Autodesk Inventor part; units mm, degrees
ref_plane "YZ Plane" through (0, 0, 0) normal (1, 0, 0) x (0, 1, 0)
ref_plane "XZ Plane" through (0, 0, 0) normal (0, 1, 0) x (-1, 0, 0)
ref_plane "XY Plane" through (0, 0, 0) normal (0, 0, 1) x (1, 0, 0)
sketch "Sketch1" plane through (0, 0, 0) normal (0, 0, 1) x (1, 0, 0)
  line L0 (0, 0) -> (37.6224, 0)
  line L1 (0, 35) -> (0, 48)
  line L2 (0, 48) -> (12.1, 50)
  line L3 (12.1, 50) -> (13.1, 50)
  line L4 (0, 35) -> (11, 34.0376)
  line L5 (11, 34.0376) -> (11, 8)
  line L6 (11, 8) -> (-1, 8)
  line L7 (-1, 8) -> (-1, 0)
  line L8 (13.1, 50) -> (13.1, 0)
  line L9 (-1, 0) -> (13.1, 0)
  line L10 (26.2, 35) -> (26.2, 48)
  line L11 (26.2, 48) -> (14.1, 50)
  line L12 (14.1, 50) -> (13.1, 50)
  line L13 (26.2, 35) -> (15.2, 34.0376)
  line L14 (15.2, 34.0376) -> (15.2, 8)
  line L15 (15.2, 8) -> (27.2, 8)
  line L16 (27.2, 8) -> (27.2, 0)
  line L17 (27.2, 0) -> (13.1, 0)
  point P0 (26.2, 0)
  dimension "d0" = 100
  dimension "d2" = 1
  dimension "d3" = 13
  dimension "d4" = 13.1
  dimension "d5" = 11
  dimension "d6" = 95
  dimension "d7" = 16
  dimension "d8" = 12
  dimension "d9" = 48
revolve "Revolution1" add sketch "Sketch1" angle 360 about axis through (0, 0, 0) along (1, 0, 0)
hole "Hole1" at (27.2, 0, 0) direction (-1, 0, 0) diameter 8 end through all
fillet "Fillet1" radius 4 2 edges at (15.2, -8, 0) (11, -8, 0)
fillet "Fillet2" radius 2 2 edges at (15.2, -34.0376, 0) (11, -34.0376, 0)
properties part number "Hjul"
Build history of the part. All positions in model axes, mm. A direction names the side the tool comes from. Give positions to 0.01 mm unless a question says otherwise; leave off trailing zeros. Loops run counter-clockwise (first coordinate to the right, second up) from the corner with the lowest first, then second, coordinate; pieces in that order, holes last.
1) Band-saw the part on A-A on x = 24.5. List the corners of the cut face in (y, z), then the cut area to 3 significant figures.
Values follow:
outline: circle Ø96.56 at (0, 0); circle Ø16 at (0, 0); hole circle Ø69.7 at (0, 0); hole circle Ø8 at (0, 0)
area: 3,660 mm2
2) Two-plate mould, pull along Y, no slides. Class faces 4 (the face through (15.2, 14, 0)), 5 (the face through (0, 3.3, -35.3)), 6 (the face through (13.11, 47.69, 15.02)): released by +Y, released by -Y, zero draft, split by the parting line, or undercut.
Values follow:
face 4: undercut
face 5: zero draft
face 6: split by the parting line
3) Band-saw the part on B-B on x = 2.75. List the corners of the cut face in (y, z).
Values follow:
outline: circle Ø96.91 at (0, 0); circle Ø16 at (0, 0); hole circle Ø69.52 at (0, 0); hole circle Ø8 at (0, 0)
4) Probe line 1 along Z through (x, y) = (5.5, 0); line 2 along Z through (x, y) = (8, 0); line 3 along Y through (x, z) = (8.75, -7). List the from-to ranges inside material, lowest first.
Values follow:
line 1: z = -48.91 to -34.52, -8 to -4, 4 to 8, 34.52 to 48.91
line 2: z = -49.32 to -34.3, -8.13 to -4, 4 to 8.13, 34.3 to 49.32
line 3: y = -48.95 to -33.51, -4.65 to 4.65, 33.51 to 48.95
5) 3-axis set-ups, long thin cutter, end or side, ignore diameter. For faces 1 (the face through (2.94, -1.73, 7.81)), 2 (the face through (23.26, -1.73, -7.81)), 3 (the face through (12.903, 3.905, 0.867)): which of +Z, -Z, +X, -X, +Y, -Y reach the whole face in a straight line?
Values follow:
face 1: -X
face 2: +X
face 3: +X, -X
6) Drop flat-ended pins along their axis: P1, Ø1.5, axis at x = 19, z = 32.5, coming from the +Y side; P2, Ø2, axis at x = 14, y = -39, coming from the -Z side; P3, Ø6, axis at y = 9, z = 10, coming from the +X side. Give the stop position or say it passes through.
Values follow:
P1: stops at y = 37.59
P2: stops at z = -32.5
P3: stops at x = 15.51
